Answer from the drawing. Dimensions are ordinates in mm from the lowest x, y and z of the part. A direction names the side the tool comes from. Coordinates: 2 decimals unless noted, no trailing zeros. Write each loop counter-clockwise with the first axis right and the second up, starting at its lowest first coordinate (ties: lowest second). Pieces come first, ordered by that corner, then holes. Notation, with made-up numbers: M 28.5,23 L 60.5,23 A26 ccw 60.5,43 Z; hole C 6.5,-22.5 d6. An arc over 180 degrees is marked long. Put each result on its own line as item: value. Start each with the question number.
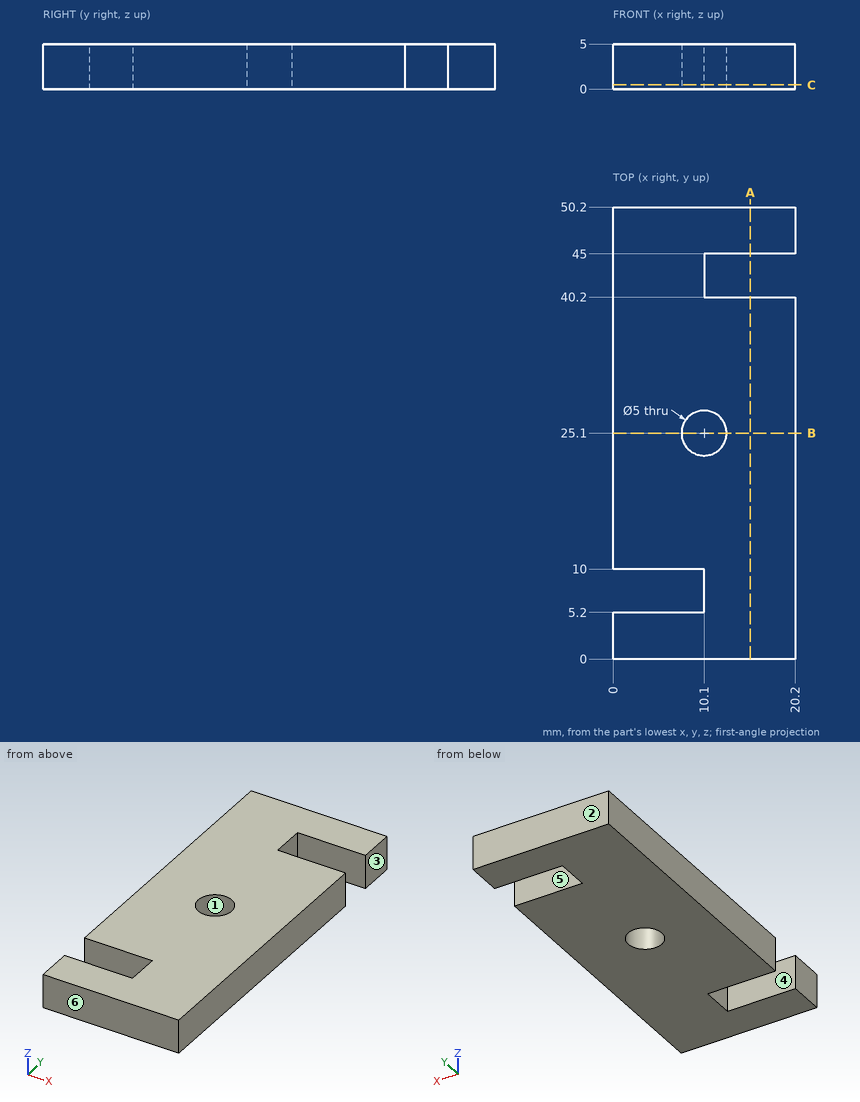
1) A cutting plane is placed at A-A on x = 15.25. Write down the section's boundary in (y, z), then the cut area to 3 significant figures.
2) A cutting plane is placed at B-B on y = 25.1. Write down the section's boundary in (x, z).
3) Given pin 1 Ø1.4 at (y, z) = (43, 1.5) entering from +X; pin 2 Ø1.4 at (y, z) = (7.5, 3) entering from -X, each flat-ended and moving along its own axis, determine where each tip first touches the part or whether it passes through.
4) For the marked faces 4, 5 and 6, determine the directions among +Z, -Z, +X, -X, +Y, -Y from which every point of the face is accessible in a straight line to the end or side of a thin tool.
5) A cutting plane is placed at C-C on z = 0.45. Write down the section's boundary in (x, y).
6) Straight lines are drawn through the part: probe 1 along Y at (x, z) = (6.75, 4.3); probe 2 along Y at (x, z) = (14, 1.45); probe 3 along Y at (x, z) = (9, 3.55) (3 decimals). For each, find the intervals that lie inside material, in ascending order.
7) Determine the mould class of the marked faces 1, 2 and 3 for opening direction Y: +Y half, -Y half, draft (parallel to the pull), parting line (faces both ways), or undercut.
Answers follow:
1. outline: M 0,0 L 40.2,0 L 40.2,5 L 0,5 Z; M 45,0 L 50.2,0 L 50.2,5 L 45,5 Z
1. area: 227 mm²
2. outline: M 0,0 L 7.6,0 L 7.6,5 L 0,5 Z; M 12.6,0 L 20.2,0 L 20.2,5 L 12.6,5 Z
3. pin 1: stops at x = 10.1
3. pin 2: stops at x = 10.1
4. face 4: +Z, -Z, -X
4. face 5: +Z, -Z, +X
4. face 6: +Z, -Z, +X, -X, -Y
5. outline: M 0,0 L 20.2,0 L 20.2,40.2 L 10.1,40.2 L 10.1,45 L 20.2,45 L 20.2,50.2 L 0,50.2 L 0,10 L 10.1,10 L 10.1,5.2 L 0,5.2 Z; hole C 10.1,25.1 d5
6. probe 1: y = 0 to 5.2, 10 to 50.2
6. probe 2: y = 0 to 40.2, 45 to 50.2
6. probe 3: y = 0 to 5.2, 10 to 22.855, 27.345 to 50.2
7. face 1: undercut
7. face 2: +Y half
7. face 3: draft
